from build123d import *

# Parameters (mm, degrees)
SKETCH1_R           = 20.0025
SKETCH1_R_2         = 14.2875
BOSS_EXTRUDE1_DEPTH = 4.572
SKETCH2_W           = 76.2
SKETCH2_H           = 50.8
SKETCH2_R           = 14.2875
BOSS_EXTRUDE2_DEPTH = 3.175
SKETCH3_R           = 15.5575
CUT_EXTRUDE1_DEPTH  = 1.651
SKETCH5_R           = 2.032
SKETCH5_R_2         = 2.54
CUT_EXTRUDE2_DEPTH  = 4.175


with BuildPart() as part:
    # Sketch1 → Boss-Extrude1 (new body)
    with BuildSketch(Plane(origin=(0, 0, 0), x_dir=(1, 0, 0), z_dir=(0, 1, 0))):
        Circle(SKETCH1_R)
        Circle(SKETCH1_R_2, mode=Mode.SUBTRACT)
    extrude(amount=BOSS_EXTRUDE1_DEPTH)

    # Sketch2 → Boss-Extrude2 (add)
    with BuildSketch(Plane.XZ):
        Rectangle(SKETCH2_W, SKETCH2_H)
        Circle(SKETCH2_R, mode=Mode.SUBTRACT)
    extrude(amount=BOSS_EXTRUDE2_DEPTH)

    # Sketch3 → Cut-Extrude1 (cut)
    with BuildSketch(Plane.XZ.offset(3.175)):
        Circle(SKETCH3_R)
    extrude(amount=-CUT_EXTRUDE1_DEPTH, mode=Mode.SUBTRACT)

    # Sketch5 → Cut-Extrude2 (cut, through all)
    with BuildSketch(Plane(origin=(0, 0, 0), x_dir=(1, 0, 0), z_dir=(0, 1, 0))):
        with Locations((-18.64995, 18.64995)):
            Circle(SKETCH5_R)
        with Locations((20.46605, 18.64995)):
            Circle(SKETCH5_R)
        with Locations((-18.64995, -20.46605)):
            Circle(SKETCH5_R)
        with Locations((20.46605, -20.46605)):
            Circle(SKETCH5_R)
        with Locations((-31.75, 15.875)):
            Circle(SKETCH5_R_2)
        with Locations((31.75, 15.875)):
            Circle(SKETCH5_R_2)
        with Locations((31.75, -15.875)):
            Circle(SKETCH5_R_2)
        with Locations((-31.75, -15.875)):
            Circle(SKETCH5_R_2)
    extrude(amount=-CUT_EXTRUDE2_DEPTH, mode=Mode.SUBTRACT)


solid = part.part
Design review of the part built by this model. Coordinates are the model's own, in mm. A direction names the side the tool comes from. Coordinates: 2 decimals unless noted, no trailing zeros. Order: outer loops, then holes, each group sorted by start corner. A loop starts at its lowest first (then second) coordinate and runs counter-clockwise, first axis right, second up. Notation, with made-up numbers: (20.25, -11) -> (51.25, -11) arc R13 ccw to (51.25, 2) -> close; hole circle Ø1 at (-7, 15). An arc over 180 degrees is marked (long way). Use one line per item in the form item = value. Start each with the question number.
(1) Add section B-B on z = 0. State the section outline as (x, y) points (1 decimal).
(2) For faces 1 (the flat face through (7, -1.524, -13)), 2 (the flat face through (-1, -2, -25.4)), 3 (the cylindrical face through (19.08, 2.25, -6.01)), list the 3-axis set-ups (+Z, -Z, +X, -X, +Y, -Y) from which the entire face can be reached by the end or side of a thin tool; tool diameter is ignored.
(3) Add section A-A on x = -31.75. State the section outline as (y, z) points (3 decimals), plus the area to 3 significant figures.
(4) Add section C-C on x = 0. State the section outline as (y, z) points (1 decimal), plus the area to 3 significant figures.
(5) For probe 1 along Z at (x, y) = (-31.75, -2.05) (3 decimals); probe 2 along X at (y, z) = (-0.5, 16); probe 3 along X at (y, z) = (2.5, 0), list the stretches that pass through material, from the lowest coordinate up.
(6) Insertion check: pin 1 (8 mm diameter, centred on x = 6, z = 12.5, fed in from +Y); pin 2 (6 mm diameter, centred on x = 31.75, z = 15.875, fed in from +Y); pin 3 (15.5 mm diameter, centred on x = 3.5, z = -6.5, fed in from -Y); pin 4 (2 mm diameter, centred on y = 2.5, z = 11.5, fed in from -X) (3 decimals). Each pin has a flat end and moves straight along its axis. Give the tip position at first contact, or say it passes through.
(7) The part is to be moulded in two halves that separate along X. For faces 4 (the cylindrical face through (31.199, -1.565, 18.355)), 5 (the flat face through (38.1, -2, 0)), 6 (the flat face through (-38.1, -2, 0)), say which applies: +X half, -X half, draft (parallel to the pull), parting line (faces both ways), or undercut.
(8) Add section D-D on y = 2.5. State the section outline as (x, z) points (1 decimal), plus the area to 3 significant figures.
Answer block:
q1.outline = (-38.1, -3.2) -> (-15.6, -3.2) -> (-15.6, -1.5) -> (-14.3, -1.5) -> (-14.3, 4.6) -> (-20, 4.6) -> (-20, 0) -> (-38.1, 0) -> close; (14.3, -1.5) -> (15.6, -1.5) -> (15.6, -3.2) -> (38.1, -3.2) -> (38.1, 0) -> (20, 0) -> (20, 4.6) -> (14.3, 4.6) -> close
q2.face_1 = -Y
q2.face_2 = -Z, +X, -X, +Y, -Y
q2.face_3 = +Y
q3.outline = (-3.175, -25.4) -> (0, -25.4) -> (0, -18.415) -> (-3.175, -18.415) -> close; (-3.175, -13.335) -> (0, -13.335) -> (0, 13.335) -> (-3.175, 13.335) -> close; (-3.175, 18.415) -> (0, 18.415) -> (0, 25.4) -> (-3.175, 25.4) -> close
q3.area = 129 mm²
q4.outline = (-3.2, -25.4) -> (0, -25.4) -> (0, -20) -> (4.6, -20) -> (4.6, -14.3) -> (-1.5, -14.3) -> (-1.5, -15.6) -> (-3.2, -15.6) -> close; (-3.2, 15.6) -> (-1.5, 15.6) -> (-1.5, 14.3) -> (4.6, 14.3) -> (4.6, 20) -> (0, 20) -> (0, 25.4) -> (-3.2, 25.4) -> close
q4.area = 119 mm²
q5.probe_1 = -25.4 to -18.415, -13.335 to 13.335, 18.415 to 25.4
q5.probe_2 = -38.1 to -34.29, -29.21 to 29.21, 34.29 to 38.1
q5.probe_3 = -20 to -14.29, 14.29 to 20
q6.pin_1 = 4.57
q6.pin_2 = 0
q6.pin_3 = -1.52
q6.pin_4 = -17.025
q7.face_4 = undercut
q7.face_5 = +X half
q7.face_6 = -X half
q8.outline = circle Ø40 at (0, 0); hole circle Ø28.6 at (0, 0)
q8.area = 616 mm²
